Work out the finished part from the listing and answer in its coordinate system (mm). A direction names the side the tool comes from. Round coordinates to 2 decimals unless told otherwise and drop trailing zeros. Order: outer loops, then holes, each group sorted by start corner. A loop starts at its lowest first (then second) coordinate and runs counter-clockwise, first axis right, second up. Notation, with made-up numbers: (78, 1.25) -> (99, 1.25) arc R22 ccw to (99, 30.25) -> close; hole circle Ø10 at (69.25, 34). An arc over 180 degrees is marked (long way). Use one line per item in the form item = value.
```python
from build123d import *

# Parameters (mm, degrees)
FILLET1_R       = 0.762
SLOT_DEPTH      = 11.006641007
SLOT_DEPTH_BACK = 11.006641007
SKETCH2_W       = 0.508
SKETCH2_H       = 4.1275


with BuildPart() as part:
    # Sketch1 → Base-Revolve (revolve)
    with BuildSketch(Plane.XY, mode=Mode.PRIVATE) as base_revolve_sk:
        with BuildLine():
            Line((0, 0.762), (4.064, 0.762))
            Line((4.064, 0.762), (4.064, 0))
            Line((4.064, 0), (1.5875, 0))
            Line((1.5875, 0), (1.5875, -5.334))
            Line((1.5875, -5.334), (2.0955, -5.334))
            Line((2.0955, -5.334), (2.0955, -6.096))
            ThreePointArc((2.0955, -6.096), (1.48174226, -7.57774226), (0, -8.1915))
            Line((0, -8.1915), (0, 0.762))
        make_face()
    revolve(base_revolve_sk.sketch.rotate(Axis((0, 0, 0), (0, -1, 0)), 180), axis=Axis((0, 0, 0), (0, -1, 0)))

    # Fillet1
    fillet1_edges = [part.edges().sort_by_distance(p)[0] for p in [
        (4.064, 0.762, 0),
    ]]
    fillet(fillet1_edges, radius=FILLET1_R - 0.0001)  # a hair under: the kernel refuses the full size

    # Sketch2 → Slot (cut, two sides: drawn at the far end of the back side and taken through both)
    with BuildSketch(Plane.XY.offset(-SLOT_DEPTH_BACK)):
        with Locations((0, -6.12775)):
            Rectangle(SKETCH2_W, SKETCH2_H)
    extrude(amount=SLOT_DEPTH + SLOT_DEPTH_BACK, mode=Mode.SUBTRACT)


solid = part.part
```
Item 1: The part is cut by section A-A, the plane y = -5.5. Give the vertices of the cut face in (x, z).
Findings:
outline = (-0.25, -2.08) -> (-0.25, 2.08) arc R2.1 ccw to start; (0.25, -2.08) arc R2.1 ccw to (0.25, 2.08) -> close
Item 2: For faces 4 (the flat face through (1.8, -5.334, 0.3)), 5 (the flat face through (0, 0.762, 0)), 6 (the flat face through (-2, 0, 0)), 7 (the cylindrical face through (2.095, -5.72, -0.043)), 8 (the flat face through (-0.254, -6, 0)), determine the directions among +Z, -Z, +X, -X, +Y, -Y from which every point of the face is accessible in a straight line to the end or side of a thin tool.
Findings:
face_4 = +X
face_5 = +Z, -Z, +X, -X, +Y
face_6 = none
face_7 = +X, -Y
face_8 = +Z, -Z, -Y
Item 3: Flat-ended cylindrical pins translate along their axes: P1, Ø3, axis at y = -2, z = -2.5, coming from the -X side; P2, Ø4.5, axis at y = -5.5, z = 0, coming from the -X side; P3, Ø1, axis at x = 2.5, z = -1.5, coming from the -Y side; P4, Ø1, axis at x = -3, y = -5.5, coming from the -Z side. Find the tip coordinate at first contact, or state that the pin passes through.
Findings:
P1 = -1.23
P2 = -2.1
P3 = 0
P4 = through
Item 4: Consider line 1 along Y through (x, z) = (2.75, -0.25); line 2 along Y through (x, z) = (0, 0.25); line 3 along X through (y, z) = (-5.5, -0.75). Determine where each line is inside the solid, lowest interval first.
Findings:
line_1 = 0 to 0.76
line_2 = -4.06 to 0.76
line_3 = -1.96 to -0.25, 0.25 to 1.96
Item 5: Determine the mould class of faces 1 (the cylindrical face through (-2.095, -5.72, 0.043)), 2 (the flat face through (0.254, -6, 0)), 3 (the flat face through (-1.72, -5.334, 0.3)) for opening direction X: released by +X, released by -X, zero draft, split by the parting line, or undercut.
Findings:
face_1 = released by -X
face_2 = undercut
face_3 = zero draft
